The listing builds one solid part. Answer for the finished solid, in the listing's coordinates (mm). A direction names the side the tool comes from. Round coordinates to 2 decimals unless told otherwise and drop trailing zeros. Write each loop counter-clockwise with the first axis right and the second up, starting at its lowest first coordinate (ties: lowest second). Pieces come first, ordered by that corner, then holes. Notation, with made-up numbers: (-1, -29) - (9, -29) arc R8 cw to (9, -22) - close; hole circle Ø3 at (-2, 83.25). An arc over 180 degrees is marked (long way). Return JSON: item names as keys, results as strings. Group by question number.
(1) This flat-tipped pin is pushed along its axis until it touches: pin 1 (4.5 mm diameter, centred on x = 182, z = -41.5, fed in from +Y). Where does it stop, or does it pass through?
(2) Determine the mould class of faces 3 (the flat face through (91, 47, -110)), 4 (the flat face through (166, 72, 2)), 5 (the flat face through (182, 54, -54)), 6 (the flat face through (91, 44, -114)) for opening direction Z: +Z half, -Z half, draft (parallel to the pull), parting line (faces both ways), or undercut.
(3) Find the intervals of material crossed by line 1 along X through (y, z) = (41, -78.5); line 2 along Z through (x, y) = (113.5, 46); line 3 along Y through (x, z) = (21.5, -94), in increasing order. Write a range as [from, to].
(4) Section C-C, the plane y = 62 is taken. Write down the section's boundary in (x, z).
(5) Section A-A, the plane y = 30 is taken. Write down the section's boundary in (x, z).
(6) Section B-B, the plane x = 169 is taken. Write down the section's boundary in (y, z).
(7) Which of the six approach directions +Z, -Z, +X, -X, +Y, -Y give full straight-line access (tool end or side, diameter ignored) to faces 1 (the flat face through (-4, 44, -56)), 2 (the flat face through (0, 47, -56))?
```python
from build123d import *

# Parameters (mm, degrees)
SKETCH1_W           = 180
SKETCH1_H           = 110
BOSS_EXTRUDE1_DEPTH = 4
SKETCH3_W           = 110
SKETCH3_H           = 54
BOSS_EXTRUDE2_DEPTH = 4
BOSS_EXTRUDE3_DEPTH = 4
SKETCH5_W           = 114
SKETCH5_H           = 89.355339059
BOSS_EXTRUDE4_DEPTH = 4
BOSS_EXTRUDE5_DEPTH = 4


with BuildPart() as part:
    # Sketch1 → Boss-Extrude1 (new body)
    with BuildSketch(Plane(origin=(0, 0, 0), x_dir=(1, 0, 0), z_dir=(0, 1, 0))):
        with Locations((90, 55)):
            Rectangle(SKETCH1_W, SKETCH1_H)
    extrude(amount=BOSS_EXTRUDE1_DEPTH)

    # Sketch3 → Boss-Extrude2 (add)
    with BuildSketch(Plane(origin=(180, 0, 0), x_dir=(0, 0, -1), z_dir=(1, 0, 0))):
        with Locations((55, 27)):
            Rectangle(SKETCH3_W, SKETCH3_H)
    extrude(amount=BOSS_EXTRUDE2_DEPTH)

    # Sketch4 → Boss-Extrude3 (add)
    with BuildSketch(Plane(origin=(0, 0, -110), x_dir=(-1, 0, 0), z_dir=(0, 0, -1))):
        Polygon((-184, 54), (-148.644660941, 89.355339059), (0, 89.355339059), (0, 4), (0, 0), (-184, 0), align=None)
    extrude(amount=BOSS_EXTRUDE3_DEPTH)

    # Sketch5 → Boss-Extrude4 (add)
    with BuildSketch(Plane.ZY):
        with Locations((-57, 44.67766953)):
            Rectangle(SKETCH5_W, SKETCH5_H)
    extrude(amount=BOSS_EXTRUDE4_DEPTH)

    # Sketch10 → Boss-Extrude5 (add)
    with BuildSketch(Plane.XY):
        Polygon((-4, 89.355339059), (148.644660941, 89.355339059), (184, 54), (184, 0), (-4, 0), align=None)
    extrude(amount=BOSS_EXTRUDE5_DEPTH)


solid = part.part
```
Working result:
{
 "1": {"pin 1": "stops at y = 54"},
 "2": {"face 3": "undercut", "face 4": "draft", "face 5": "undercut", "face 6": "-Z half"},
 "3": {"line 1": "x = [-4, 0], [180, 184]", "line 2": "z = [-114, -110], [0, 4]", "line 3": "y = [0, 4]"},
 "4": {"outline": "(-4, -114) - (176, -114) - (176, -110) - (0, -110) - (0, 0) - (176, 0) - (176, 4) - (-4, 4) - close"},
 "5": {"outline": "(-4, -114) - (184, -114) - (184, 4) - (-4, 4) - close; hole (0, -110) - (180, -110) - (180, 0) - (0, 0) - close"},
 "6": {"outline": "(0, -114) - (69, -114) - (69, -110) - (4, -110) - (4, 0) - (69, 0) - (69, 4) - (0, 4) - close"},
 "7": {"face 1": "+Z, -Z, -X, +Y, -Y", "face 2": "+Y"}
}
